Autodesk Inventor part; units mm, degrees
ref_plane "YZ Plane" through (0, 0, 0) normal (1, 0, 0) x (0, 1, 0)
ref_plane "XZ Plane" through (0, 0, 0) normal (0, 1, 0) x (-1, 0, 0)
ref_plane "XY Plane" through (0, 0, 0) normal (0, 0, 1) x (1, 0, 0)
sketch "Sketch2" plane through (0, 0, 0) normal (0, 0, 1) x (1, 0, 0)
  line L0 (0, 0) -> (-9.9, 0)
  line L1 (-4.95, 0) -> (-4.95, 2.5)
  line L2 (-4.95, 0) -> (-2.45, 0) construction
  circle A0 centre (-4.95, 5) radius 2.5
  line L3 (-4.95, 7.5) -> (32.05, 7.5) construction
  line L4 (0, 0) -> (-9.9, 0)
  line L5 (0, 0) -> (-9.9, 0)
  line L6 (-4.95, 7.5) -> (66.05, 7.5) construction
  line L7 (-4.95, 7.5) -> (70.05, 7.5) construction
  line L8 (0, 0) -> (-9.9, 0)
  line L9 (-9.9, 0) -> (-9.9, 82.5)
  line L10 (0, 82.5) -> (0, 0)
  line L11 (-4.95, 7.5) -> (74.05, 7.5) construction
  line L12 (-9.9, 86.5) -> (0, 86.5)
  line L13 (0, 86.5) -> (0, 82.5)
  line L14 (-9.9, 82.5) -> (-9.9, 86.5)
  dimension "d35" = 5
  dimension "d33" = 2.5
  dimension "d34" = 90
  dimension "d48" = 9.9
extrude "Extrusion7" add sketch "Sketch2" along normal blind 5
properties part number "Cube_Holder_SB_V1_(71mm)"
Build history of the part. All positions in model axes, mm. Coordinates: 2 decimals unless noted, no trailing zeros. Order: outer loops, then holes, each group sorted by start corner. A loop starts at its lowest first (then second) coordinate and runs counter-clockwise, first axis right, second up.
Item 1: Drill centre lines: L1, parallel to X at y = 5, z = 1.7; L2, parallel to Y at x = -4.95, z = 1.6; L3, parallel to Y at x = -7, z = 2.85. Where is each one in solid material? Low to high.
Filled in:
L1: x = -9.9 to -7.45, -2.45 to 0
L2: y = 0 to 2.5, 7.5 to 86.5
L3: y = 0 to 3.57, 6.43 to 86.5
Item 2: Saw through at B-B on y = 5. List the corners of the cut face in (x, z), then the cut area to 3 significant figures.
Filled in:
outline: (-9.9, 0) - (-7.45, 0) - (-7.45, 5) - (-9.9, 5) - close; (-2.45, 0) - (0, 0) - (0, 5) - (-2.45, 5) - close
area: 24.5 mm2
Item 3: Saw through at C-C on z = 2.95. List the corners of the cut face in (x, y).
Filled in:
outline: (-9.9, 0) - (0, 0) - (0, 86.5) - (-9.9, 86.5) - close; hole circle Ø5 at (-4.95, 5)
Item 4: Saw through at A-A on x = -4.95. List the corners of the cut face in (y, z), then the cut area to 4 significant figures.
Filled in:
outline: (0, 0) - (2.5, 0) - (2.5, 5) - (0, 5) - close; (7.5, 0) - (86.5, 0) - (86.5, 5) - (7.5, 5) - close
area: 407.5 mm2
Item 5: Mould opens along Y. For faces 1 (the flat face through (-5, 0, 2)), 2 (the flat face through (-5, 44, 5)), 3 (the cylindrical face through (-2.565, 4.249, 2.465)) say: released by +Y, released by -Y, zero draft, split by the parting line, or undercut.
Filled in:
face 1: released by -Y
face 2: zero draft
face 3: undercut
